Source: CAD feature listing. Evaluate the final solid. Frame: model axes, mm. Give positions to 0.01 mm unless a question says otherwise; leave off trailing zeros. Order: outer loops, then holes, each group sorted by start corner. A loop starts at its lowest first (then second) coordinate and runs counter-clockwise, first axis right, second up. Notation, with made-up numbers: (-33, 68.25) - (-12, 68.25) arc R31 cw to (-12, 97.25) - close; hole circle Ø9 at (79.25, 33). An arc over 180 degrees is marked (long way). Answer as CSV lines item,"result".
```python
from build123d import *

# Parameters (mm, degrees)
F2_T = -5


# Not quite as in the source:
# - a fillet or chamfer that OpenCascade refuses, or shapes differently, is made with other operations: its cross-section is extruded or revolved along the edge and cut away or added
# - a feature of the source that left no trace in its solid (it failed there, or was rolled back) is left out


with BuildPart() as f1:
    # F0 (on Front) → F1 (revolve)
    with BuildSketch(Plane.XZ):
        Polygon((0, 210), (0, 0), (210, 0), align=None)
    revolve(axis=Axis((0, 0, 105), (0, 0, 1)))

    # F2
    f2_openings = [f1.faces().sort_by_distance(p)[0] for p in [
        (0, 0, 0),
    ]]
    offset(amount=F2_T, openings=f2_openings)

    # F3: fillet of radius 5 on 1 edges, made by hand

    # F3_s1 → F3_t2 (revolve, cut)
    with BuildSketch(Plane.XZ):
        with BuildLine():
            ThreePointArc((202.9289321881, 7.0710678119), (204.3933982822, 3.5355339059), (202.9289321881, 0))
            Line((202.9289321881, 0), (210, 0))
            Line((210, 0), (202.9289321881, 7.0710678119))
        make_face()
    revolve(axis=Axis((0, 0, 0), (0, 0, 1)), mode=Mode.SUBTRACT)


solid = f1.part
```
(1) Cut plane A-A (z = 133.5). Return loops of the section in (x, y).
Completed:
outline,"circle Ø153 at (0, 0); hole circle Ø138.86 at (0, 0)"
(2) Contact query for flat-ended pins moving along their axis: pin 1 (1 mm diameter, centred on x = -51.5, y = 119.5, fed in from -Z); pin 2 (8 mm diameter, centred on x = 66, z = 33, fed in from +Y); pin 3 (3 mm diameter, centred on x = -162, y = -36.5, fed in from +Z). Output: stop coordinate, or through.
Completed:
pin 1,"z = 72.3"
pin 2,"y = 168.81"
pin 3,"z = 45.44"
(3) Cut plane B-B (z = 99.5). Return loops of the section in (x, y), then the cut area to 3 significant figures.
Completed:
outline,"circle Ø221 at (0, 0); hole circle Ø206.86 at (0, 0)"
area,"4,750 mm²"
(4) Mould query, pull axis Y, two halves, no side actions, for faces 1 (the conical face through (52.41, 16.51, 147.98)), 2 (the conical face through (-44, -33, 155)). Classes: released by +Y, released by -Y, zero draft, split by the parting line, or undercut.
Completed:
face 1,"undercut"
face 2,"split by the parting line"
(5) Ray query, line 1 (Y direction, x = 104.5, z = 46); line 2 (X direction, y = 58, z = 48.5); line 3 (Y direction, x = -28, z = 134.5). Return the intervals inside material, ascending. Write a range as from..to.
Completed:
line 1,"-126.4..-117.07, 117.07..126.4"
line 2,"-150.73..-143.12, 143.12..150.73"
line 3,"-70.12..-62.44, 62.44..70.12"
